Geometry check sheet. Reference: drawing and pictorial views, mm from the part's lowest x, y, z. Coordinates: 2 decimals unless noted, no trailing zeros. Loops run counter-clockwise (first coordinate to the right, second up) from the corner with the lowest first, then second, coordinate; pieces in that order, holes last. Notation, with made-up numbers: (87, 34) - (92, 34) arc R21 cw to (92, 47) - close; hole circle Ø3 at (42.5, -15.75). An arc over 180 degrees is marked (long way). Use a Markdown table: item, result. Add a question column.
1) Thickness scan on line 1 (X direction, y = 0.6, z = 5); line 2 (Z direction, x = 36, y = 1.4); line 3 (X direction, y = 0.4, z = 4.25). Record the ranges inside material, lowest first.
2) Sectioned sample at D-D, the plane z = 8.75. Enter the section's corners in (x, y), then the cut area to 3 significant figures.
3) Sectioned sample at C-C, the plane z = 5. Enter the section's corners in (x, y), then the cut area to 3 significant figures.
4) Sectioned sample at B-B, the plane y = 0.75. Enter the section's corners in (x, z), then the cut area to 3 significant figures.
5) Go/stop test with a flat-tipped pin: P1, Ø1.8, axis at x = 36, z = 5, coming from the +Y side. Record where the tip stops, or that it passes through.
6) Sectioned sample at A-A, the plane x = 4. Enter the section's corners in (y, z), then the cut area to 3 significant figures.
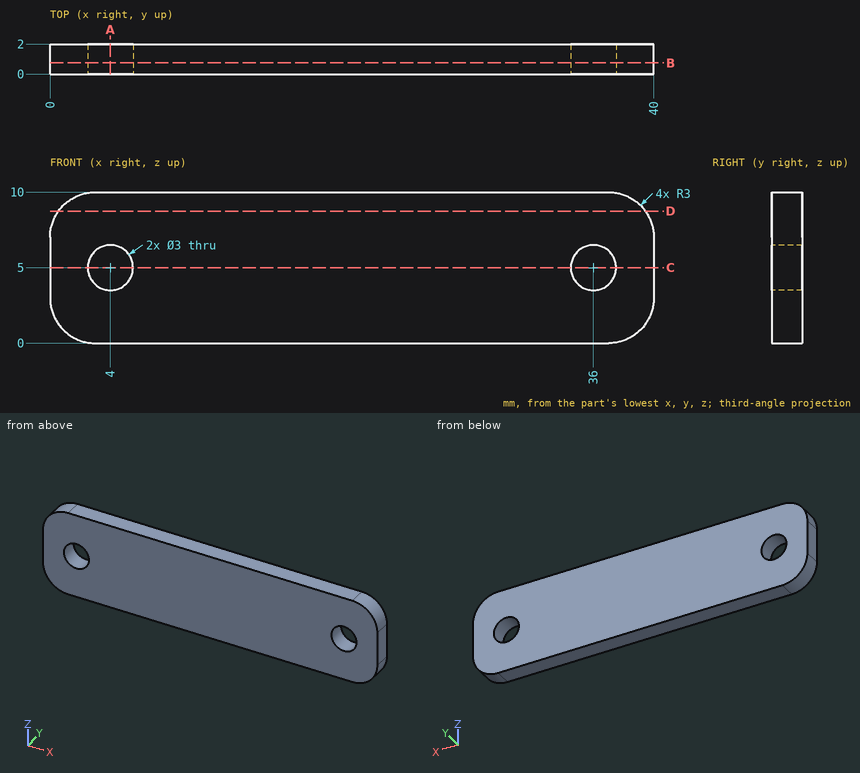
Solved:
| question | item | result |
|---|---|---|
| 1 | line 1 | x = 0 to 2.5, 5.5 to 34.5, 37.5 to 40 |
| 1 | line 2 | z = 0 to 3.5, 6.5 to 10 |
| 1 | line 3 | x = 0 to 2.7, 5.3 to 34.7, 37.3 to 40 |
| 2 | outline | (0.56, 0) - (39.44, 0) - (39.44, 2) - (0.56, 2) - close |
| 2 | area | 77.7 mm2 |
| 3 | outline | (0, 0) - (2.5, 0) - (2.5, 2) - (0, 2) - close; (5.5, 0) - (34.5, 0) - (34.5, 2) - (5.5, 2) - close; (37.5, 0) - (40, 0) - (40, 2) - (37.5, 2) - close |
| 3 | area | 68.0 mm2 |
| 4 | outline | (0, 3) arc R3 ccw to (3, 0) - (37, 0) arc R3 ccw to (40, 3) - (40, 7) arc R3 ccw to (37, 10) - (3, 10) arc R3 ccw to (0, 7) - close; hole circle Ø3 at (4, 5); hole circle Ø3 at (36, 5) |
| 4 | area | 378 mm2 |
| 5 | P1 | passes through |
| 6 | outline | (0, 0) - (2, 0) - (2, 3.5) - (0, 3.5) - close; (0, 6.5) - (2, 6.5) - (2, 10) - (0, 10) - close |
| 6 | area | 14.0 mm2 |
